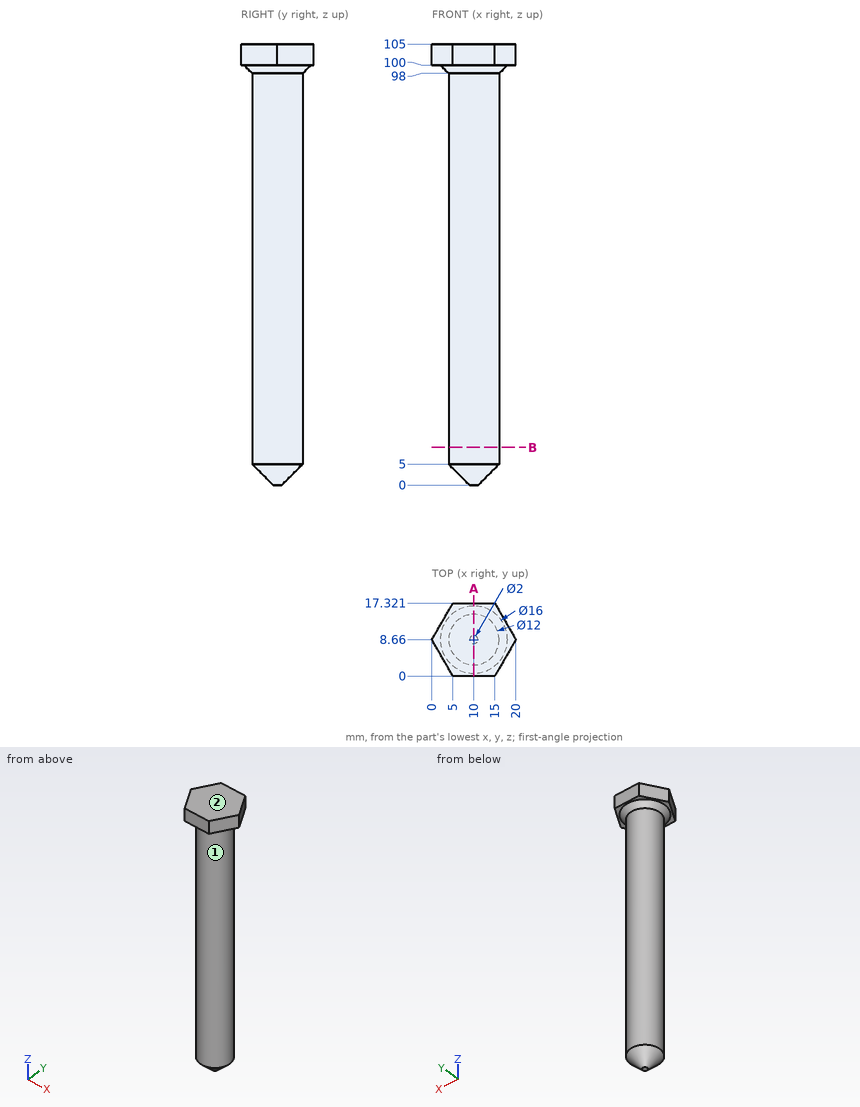
Check sheet for the drawn part. Datum: minimum x, y, z corner. Units: mm. A direction names the side the tool comes from. Round coordinates to 2 decimals unless told otherwise and drop trailing zeros. Write each loop counter-clockwise with the first axis right and the second up, starting at its lowest first coordinate (ties: lowest second). Pieces come first, ordered by that corner, then holes. Notation, with made-up numbers: (60.5, 57.25) -> (111.5, 57.25) arc R23 ccw to (111.5, 83.25) -> close; hole circle Ø5 at (73, 78.25). An arc over 180 degrees is marked (long way). Write each question's results on one line, items separated by ' | '.
Q1. Sectioned sample at B-B, the plane z = 9. Record the boundary of the cut face in (x, y).
Derived:
outline: circle Ø12 at (10, 8.66)
Q2. Sectioned sample at A-A, the plane x = 10. Record the boundary of the cut face in (y, z), and give its area (3 significant figures).
Derived:
outline: (0, 100) -> (0.66, 100) -> (2.66, 98) -> (2.66, 5) -> (7.66, 0) -> (9.66, 0) -> (14.66, 5) -> (14.66, 98) -> (16.66, 100) -> (17.32, 100) -> (17.32, 105) -> (0, 105) -> close | area: 1,270 mm²
Q3. Thickness scan on probe 1 along X at (y, z) = (8.75, 73); probe 2 along Z at (x, y) = (19, 9.25); probe 3 along X at (y, z) = (3.25, 25) (1 decimal). Record the ranges inside material, lowest first.
Derived:
probe 1: x = 4 to 16 | probe 2: z = 100 to 105 | probe 3: x = 7.4 to 12.6
Q4. Access from +Z, -Z, +X, -X, +Y, -Y to the whole of each face (thin tool, end or side, straight path). Record for the marked faces 1 and 2.
Derived:
face 1: -Z | face 2: +Z, +X, -X, +Y, -Y
Q5. Go/stop test with flat-tipped pins: pin 1 Ø1.5 at (x, z) = (10, 31) entering from -Y; pin 2 Ø6 at (x, z) = (9.5, 86) entering from +Y; pin 3 Ø6 at (y, z) = (9.5, 92) entering from +X. Record where each tip stops, or that it passes through.
Derived:
pin 1: stops at y = 2.66 | pin 2: stops at y = 14.66 | pin 3: stops at x = 16
